Check sheet for the drawn part. Datum: minimum x, y, z corner. Units: mm. Coordinates: 2 decimals unless noted, no trailing zeros. Loops run counter-clockwise (first coordinate to the right, second up) from the corner with the lowest first, then second, coordinate; pieces in that order, holes last.
Q1. Sectioned sample at A-A (x = 9.75). Enter the section's corners in (y, z).
Q2. Sectioned sample at D-D (y = 0.8). Enter the section's corners in (x, z), then the cut area to 3 significant figures.
Q3. Sectioned sample at C-C (z = 3.25). Enter the section's corners in (x, y).
Q4. Sectioned sample at B-B (z = 21). Enter the section's corners in (x, y).
Q5. Material ranges on probe 1 along Z at (x, y) = (9.75, 1.95); probe 2 along X at (y, z) = (2, 21); probe 3 along X at (y, z) = (1.2, 21), recorded low to high.
Q6. Go/stop test with flat-tipped pins: P1, Ø0.8, axis at x = 68, y = 1, coming from the +Z side; P2, Ø1, axis at x = 68, z = 19, coming from the +Y side. Record where each tip stops, or that it passes through.
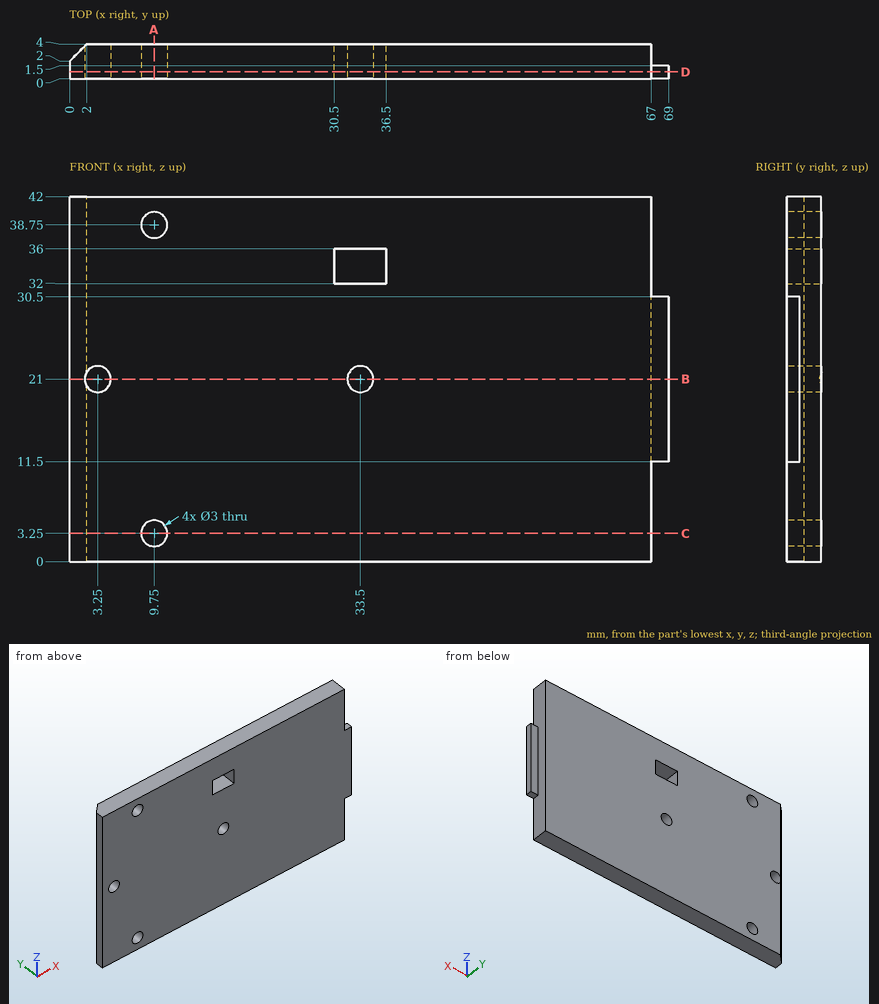
Geometry check:
1. outline: (0, 0) - (4, 0) - (4, 1.75) - (0, 1.75) - close; (0, 4.75) - (4, 4.75) - (4, 37.25) - (0, 37.25) - close; (0, 40.25) - (4, 40.25) - (4, 42) - (0, 42) - close
2. outline: (0, 0) - (67, 0) - (67, 11.5) - (69, 11.5) - (69, 30.5) - (67, 30.5) - (67, 42) - (0, 42) - close; hole circle Ø3 at (3.25, 21); hole circle Ø3 at (9.75, 3.25); hole circle Ø3 at (9.75, 38.75); hole (30.5, 32) - (36.5, 32) - (36.5, 36) - (30.5, 36) - close; hole circle Ø3 at (33.5, 21)
2. area: 2,800 mm2
3. outline: (0, 0) - (8.25, 0) - (8.25, 4) - (2, 4) - (0, 2) - close; (11.25, 0) - (67, 0) - (67, 4) - (11.25, 4) - close
4. outline: (0, 0) - (1.75, 0) - (1.75, 3.75) - (0, 2) - close; (4.75, 0) - (32, 0) - (32, 4) - (4.75, 4) - close; (35, 0) - (69, 0) - (69, 1.5) - (67, 1.5) - (67, 4) - (35, 4) - close
5. probe 1: z = 0 to 1.75, 4.75 to 37.25, 40.25 to 42
5. probe 2: x = 0 to 1.75, 4.75 to 32, 35 to 67
5. probe 3: x = 0 to 1.75, 4.75 to 32, 35 to 69
6. P1: stops at z = 30.5
6. P2: stops at y = 1.5
